from build123d import *

# Parameters (mm, degrees)
F0_R     = 14
F1_DEPTH = 3
F3_DEPTH = 3
F4_SCALE = 0.7143


# Not quite as in the source:
# - a feature names something its author has since deleted; it is built from what else it names


with BuildPart() as f1:
    # F0 (on Top) → F1 (new body)
    with BuildSketch(Plane.XY):
        Circle(F0_R)
    extrude(amount=F1_DEPTH)

    # F2 (on face) → F3 (join)
    with BuildSketch(Plane.XY.offset(3)):
        Polygon((0, 3.5), (2.5, 3.5), (0, 7.8301270189), (-2.5, 3.5), align=None)
        Polygon((-1.7810889132, -3.9150635095), (-3.0310888244, -1.7500001539), (-4.2810889132, 0.4150635095), (-6.7810889132, -3.9150635095), align=None)
        Polygon((4.2810889132, 0.4150635095), (3.0310888244, -1.7500001539), (1.7810889132, -3.9150635095), (6.7810889132, -3.9150635095), align=None)
        Polygon((-8.1317279836, 4.5961940777), (-6.3639610341, 6.3639610272), (-4.5961940777, 8.1317279836), (-9.4258232092, 9.4258232092), align=None)
        Polygon((0, 9), (2.5, 9), (0, 13.3301270189), (-2.5, 9), align=None)
        Polygon((4.5961940777, 8.1317279836), (6.3639610512, 6.3639610102), (8.1317279836, 4.5961940777), (9.4258232092, 9.4258232092), align=None)
        Polygon((9, 2.5), (9, 0), (9, -2.5), (13.3301270189, 0), align=None)
        Polygon((8.1317279836, -4.5961940777), (6.3639610307, -6.3639610307), (4.5961940777, -8.1317279836), (9.4258232092, -9.4258232092), align=None)
        Polygon((2.5, -9), (0, -9), (-2.5, -9), (0, -13.3301270189), align=None)
        Polygon((-4.5961940777, -8.1317279836), (-6.3639610486, -6.3639610128), (-8.1317279836, -4.5961940777), (-9.4258232092, -9.4258232092), align=None)
        Polygon((-9, -2.5), (-9, 0), (-9, 2.5), (-13.3301270189, 0), align=None)
    extrude(amount=F3_DEPTH)


with BuildPart() as f1_1:
    # F4: moved
    add(f1.part.scale(F4_SCALE))


solid = f1_1.part
Read the model definition and answer for the solid it produces. Units are mm, in the model's axes. A direction names the side the tool comes from. Give positions to 0.01 mm unless a question says otherwise; leave off trailing zeros. Write each loop counter-clockwise with the first axis right and the second up, starting at its lowest first coordinate (ties: lowest second). Pieces come first, ordered by that corner, then holes. Notation, with made-up numbers: (-12, 12.25) -> (9, 12.25) arc R32 ccw to (9, 43.25) -> close; hole circle Ø6 at (-16, 89.25). An arc over 180 degrees is marked (long way). Answer as a JSON object with one key per item and string values. Group by question number.
1) The mould has two halves that part along X. Classify faces 4 (the cylindrical face through (-2.17, -9.76, 1.06)), 5 (the flat face through (-6.264, -4.984, 3.199)), 6 (the flat face through (-3.94, -1.23, 3.2)), 7 (the flat face through (-3, -2.797, 3)): +X half, -X half, draft (parallel to the pull), parting line (faces both ways), or undercut.
2) Find section A-A (z = 1.7). Write down the section's boundary in (x, y), and give its area (3 significant figures).
3) Find section D-D (y = 4). Write down the section's boundary in (x, z).
4) Consider L1, parallel to X at y = 5.25, z = 2.8; L2, parallel to Y at x = 0.75, z = 4.15; L3, parallel to X at y = 4, z = 3.9. Determine where each line is inside the solid, lowest interval first. Write a range as from..to.
5) Each of these flat-tipped pins is pushed along its axis until it touches: P1, Ø2.5, axis at y = 0.5, z = 3.5, coming from the +X side; P2, Ø1.7, axis at x = 1, z = 3.5, coming from the +Y side; P3, Ø1.1, axis at x = -0.5, z = 3, coming from the -Y side. Where does it stop, or does it pass through?
6) Find section C-C (y = -4.25). Write down the section's boundary in (x, z).
7) Find section B-B (x = 8). Write down the section's boundary in (y, z), and give its area (3 significant figures).
8) A tool of negligible diameter and unlimited length cuts with its end or side. For faces 1 (the flat face through (3, -2.797, 3)), 2 (the flat face through (-0.88, 4.07, 3.2)), 3 (the flat face through (-5.032, -6.277, 3.199)), from which of +Z, -Z, +X, -X, +Y, -Y can it reach the whole face along a straight path? Write none if from no direction.
Values follow:
{
 "1": {"face 4": "parting line", "face 5": "-X half", "face 6": "undercut", "face 7": "draft"},
 "2": {"outline": "circle Ø20 at (0, 0)", "area": "314 mm2"},
 "3": {"outline": "(-9.17, 0) -> (9.17, 0) -> (9.17, 2.14) -> (6, 2.14) -> (6, 4.29) -> (5.09, 4.29) -> (5.09, 2.14) -> (0.92, 2.14) -> (0.92, 4.29) -> (-0.92, 4.29) -> (-0.92, 2.14) -> (-5.09, 2.14) -> (-5.09, 4.29) -> (-6, 4.29) -> (-6, 2.14) -> (-9.17, 2.14) -> close"},
 "4": {"L1": "x = -6.34..-3.84, -0.2..0.2, 3.84..6.34", "L2": "y = -8.22..-6.43, 2.5..4.29, 6.43..8.22", "L3": "x = -6..-5.09, -0.92..0.92, 5.09..6"},
 "5": {"P1": "stops at x = 9.52", "P2": "stops at y = 9.26", "P3": "stops at y = -9.52"},
 "6": {"outline": "(-9.05, 0) -> (9.05, 0) -> (9.05, 2.14) -> (6.07, 2.14) -> (6.07, 4.29) -> (4.84, 4.29) -> (4.84, 2.14) -> (-4.84, 2.14) -> (-4.84, 4.29) -> (-6.07, 4.29) -> (-6.07, 2.14) -> (-9.05, 2.14) -> close"},
 "7": {"outline": "(-6, 0) -> (6, 0) -> (6, 2.14) -> (0.88, 2.14) -> (0.88, 4.29) -> (-0.88, 4.29) -> (-0.88, 2.14) -> (-6, 2.14) -> close", "area": "29.5 mm2"},
 "8": {"face 1": "+Z, +X, -X", "face 2": "+Z", "face 3": "+Z, -Y"}
}
